Could you check a few things on this model? Use its own coordinates, in mm. Coordinates: 2 decimals unless noted, no trailing zeros. Order: outer loops, then holes, each group sorted by start corner. A loop starts at its lowest first (then second) coordinate and runs counter-clockwise, first axis right, second up. Notation, with made-up numbers: (74.5, 31) - (87.5, 31) arc R18 cw to (87.5, 35) - close; hole circle Ø6 at (54, 67). An arc over 180 degrees is marked (long way). One line per item, written item: value.
from build123d import *

# Parameters (mm, degrees)
SKETCH1_W               = 25.4
SKETCH1_H               = 6.35
BOSS_EXTRUDE1_DEPTH     = 11.43
CHAMFER2_SIZE           = 5.08
F_1_4_20_TAPPED_HOLE1_D = 5.1054


with BuildPart() as part:
    # Sketch1 → Boss-Extrude1 (new body)
    with BuildSketch(Plane.XY):
        Rectangle(SKETCH1_W, SKETCH1_H)
    extrude(amount=BOSS_EXTRUDE1_DEPTH)

    # Chamfer2
    chamfer2_edges = [part.edges().sort_by_distance(p)[0] for p in [
        (-12.7, 3.175, 5.715),
        (12.7, 3.175, 5.715),
    ]]
    chamfer(chamfer2_edges, length=CHAMFER2_SIZE)

    # 1/4-20 Tapped Hole1 (through all)
    with Locations(Plane(origin=(0, 3.175, 0), x_dir=(-1, 0, 0), z_dir=(0, 1, 0))):
        with Locations((0, 5.715)):
            Hole(F_1_4_20_TAPPED_HOLE1_D / 2)


solid = part.part
Item 1: I'm going to push flat-ended pins straight in: pin 1 Ø4 at (x, z) = (0, 5.715) entering from -Y; pin 2 Ø2 at (y, z) = (0.5, 5) entering from -X (3 decimals). Where does each tip first touch, or does it pass through?
Conclusion:
pin 1: through
pin 2: x = -11.295
Item 2: I want a section at A-A on z = 5.25. Please give me the cut outline in (x, y) (3 decimals).
Conclusion:
outline: (-12.7, -3.175) - (-2.51, -3.175) - (-2.51, 3.175) - (-7.62, 3.175) - (-12.7, -1.905) - close; (2.51, -3.175) - (12.7, -3.175) - (12.7, -1.905) - (7.62, 3.175) - (2.51, 3.175) - close
Item 3: Thinking about a two-plate mould opening in X: for faces 1 (the face through (-10.124, 0.671, 5.635)), 2 (the face through (10.124, 0.671, 5.635)), 3 (the face through (0, 3.175, 3)), 4 (the face through (2.435, -0.044, 6.482)), which applies, pulls with the +X half, pulls with the -X half, needs draft (parallel to the pull), parting line crosses it, or undercut?
Conclusion:
face 1: pulls with the -X half
face 2: pulls with the +X half
face 3: needs draft
face 4: undercut
Item 4: I want a section at B-B on x = 0. Please give me the cut outline in (y, z) (3 decimals).
Conclusion:
outline: (-3.175, 0) - (3.175, 0) - (3.175, 3.162) - (-3.175, 3.162) - close; (-3.175, 8.268) - (3.175, 8.268) - (3.175, 11.43) - (-3.175, 11.43) - close
Item 5: I want a section at C-C on y = -1.25. Please give me the cut outline in (x, z) (3 decimals).
Conclusion:
outline: (-12.045, 0) - (12.045, 0) - (12.045, 11.43) - (-12.045, 11.43) - close; hole circle Ø5.105 at (0, 5.715)
Item 6: If I drill on probe 1 along Z at (x, y) = (0, 0.5); probe 2 along X at (y, z) = (1.5, 7) (3 decimals); probe 3 along X at (y, z) = (-1.5, 4) (3 decimals), over which ranges is the centre line in solid material (lowest first)?
Conclusion:
probe 1: 0 to 3.16, 8.27 to 11.43
probe 2: -9.295 to -2.206, 2.206 to 9.295
probe 3: -12.295 to -1.891, 1.891 to 12.295
Item 7: I want a section at D-D on z = 2.75. Please give me the cut outline in (x, y) (3 decimals), then the cut area to 3 significant figures.
Conclusion:
outline: (-12.7, -3.175) - (12.7, -3.175) - (12.7, -1.905) - (7.62, 3.175) - (-7.62, 3.175) - (-12.7, -1.905) - close
area: 135 mm²
